Build history of the part. All positions in model axes, mm. Give positions to 0.01 mm unless a question says otherwise; leave off trailing zeros. Write each loop counter-clockwise with the first axis right and the second up, starting at its lowest first coordinate (ties: lowest second). Pieces come first, ordered by that corner, then holes. Notation, with made-up numbers: (36.25, 54.25) -> (95.25, 54.25) arc R26 ccw to (95.25, 92.25) -> close; hole circle Ø5 at (-6, -20). An arc over 180 degrees is marked (long way). Put each result on its own line as item: value.
from build123d import *

# Parameters (mm, degrees)
F0_R     = 9.95
F1_DEPTH = 3


with BuildPart() as f1:
    # F0 (on Top) → F1 (new body)
    with BuildSketch(Plane.XY):
        with BuildLine():
            ThreePointArc((7.205074, 13.15625), (0, 44.5), (-7.205074, 13.15625))
            ThreePointArc((-7.205074, 13.15625), (-10.486295, 10.725559), (-12.990381, 7.5))
            ThreePointArc((-12.990381, 7.5), (-14.531754, 3.718619), (-14.996184, -0.338348))
            ThreePointArc((-14.996184, -0.338348), (-38.53813, -22.25), (-7.79111, -12.817902))
            ThreePointArc((-7.79111, -12.817902), (-4.045459, -14.444177), (0, -15))
            ThreePointArc((0, -15), (4.045459, -14.444177), (7.79111, -12.817902))
            ThreePointArc((7.79111, -12.817902), (38.53813, -22.25), (14.996184, -0.338348))
            ThreePointArc((14.996184, -0.338348), (14.531754, 3.718619), (12.990381, 7.5))
            ThreePointArc((12.990381, 7.5), (10.486295, 10.725559), (7.205074, 13.15625))
        make_face()
        with Locations((-24.248711, -14)):
            Circle(F0_R, mode=Mode.SUBTRACT)
        with BuildLine():
            ThreePointArc((0, 11), (5.5, 9.526279), (9.526279, 5.5))
            ThreePointArc((9.526279, 5.5), (9.526279, -5.5), (0, -11))
            ThreePointArc((0, -11), (-9.526279, -5.5), (-9.526279, 5.5))
            ThreePointArc((-9.526279, 5.5), (-5.5, 9.526279), (0, 11))
        make_face(mode=Mode.SUBTRACT)
        with Locations((24.248711, -14)):
            Circle(F0_R, mode=Mode.SUBTRACT)
        with BuildLine():
            ThreePointArc((9.95, 28), (7.035712, 20.964288), (0, 18.05))
            ThreePointArc((0, 18.05), (-7.035712, 35.035712), (9.95, 28))
        make_face(mode=Mode.SUBTRACT)
    extrude(amount=F1_DEPTH)


solid = f1.part
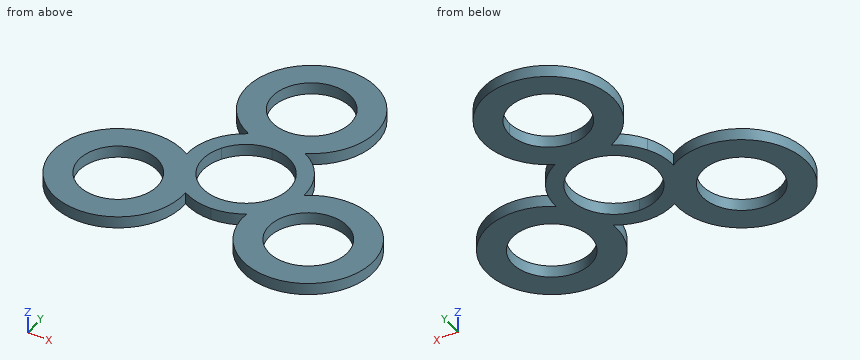
1) Slice it at B-B (x = -6). Write the cut outline in (y, z).
Filled sheet:
outline: (-13.75, 0) -> (-9.22, 0) -> (-9.22, 3) -> (-13.75, 3) -> close; (9.22, 0) -> (20.06, 0) -> (20.06, 3) -> (9.22, 3) -> close; (35.94, 0) -> (43.37, 0) -> (43.37, 3) -> (35.94, 3) -> close
2) Slice it at A-A (y = 35.5). Write the cut outline in (x, z), plus the area to 3 significant figures.
Filled sheet:
outline: (-14.7, 0) -> (-6.54, 0) -> (-6.54, 3) -> (-14.7, 3) -> close; (6.54, 0) -> (14.7, 0) -> (14.7, 3) -> (6.54, 3) -> close
area: 49.0 mm2
3) Slice it at C-C (z = 0.75). Write the cut outline in (x, y).
Filled sheet:
outline: (-15, -0.34) arc R16.5 ccw (long way) to (-7.79, -12.82) arc R15 ccw to (0, -15) arc R15 ccw to (7.79, -12.82) arc R16.5 ccw (long way) to (15, -0.34) arc R15 ccw to (12.99, 7.5) arc R15 ccw to (7.21, 13.16) arc R16.5 ccw (long way) to (-7.21, 13.16) arc R15 ccw to (-12.99, 7.5) arc R15 ccw to start; hole circle Ø19.9 at (-24.25, -14); hole (-9.53, 5.5) arc R11 ccw (long way) to (9.53, 5.5) arc R11 ccw to (0, 11) arc R11 ccw to start; hole (0, 18.05) arc R9.95 ccw to (9.95, 28) arc R9.95 ccw (long way) to start; hole circle Ø19.9 at (24.25, -14)
4) Pin check, flat tip, straight feed: pin 1 (1 mm diameter, centred on x = 2, z = 2.5, fed in from +Y). Stop position of the tip, or through.
Filled sheet:
pin 1: y = 44.43
5) Wall check: L1, parallel to X at y = 28, z = 1.65; L2, parallel to Y at x = 24.5, z = 2.1; L3, parallel to Y at x = -3.5, z = 2.05. Give the ranges that are in metal, low to high.
Filled sheet:
L1: -16.5 to -9.95, 9.95 to 16.5
L2: -30.5 to -23.95, -4.05 to 2.5
L3: -14.59 to -10.43, 10.43 to 18.69, 37.31 to 44.12
6) Slice it at D-D (x = 19.5). Write the cut outline in (y, z).
Filled sheet:
outline: (-29.8, 0) -> (-22.74, 0) -> (-22.74, 3) -> (-29.8, 3) -> close; (-5.26, 0) -> (1.8, 0) -> (1.8, 3) -> (-5.26, 3) -> close
